```python
from build123d import *

# Parameters (mm, degrees)
SKETCH1_R           = 5
BOSS_EXTRUDE1_DEPTH = 2
SKETCH2_R           = 4.3
BOSS_EXTRUDE2_DEPTH = 3
CHAMFER1_SIZE       = 1
CHAMFER1_SIZE2      = 0.577350269


with BuildPart() as part:
    # Sketch1 → Boss-Extrude1 (new body)
    with BuildSketch(Plane(origin=(0, 0, 0), x_dir=(1, 0, 0), z_dir=(0, 1, 0))):
        Circle(SKETCH1_R)
    extrude(amount=BOSS_EXTRUDE1_DEPTH)

    # Sketch2 → Boss-Extrude2 (add)
    with BuildSketch(Plane(origin=(0, 2, 0), x_dir=(1, 0, 0), z_dir=(0, 1, 0))):
        Circle(SKETCH2_R)
    extrude(amount=BOSS_EXTRUDE2_DEPTH)

    # Chamfer1
    chamfer1_edges = [part.edges().sort_by_distance(p)[0] for p in [
        (-4.3, 5, 0),
    ]]
    chamfer1_side = [part.faces().sort_by_distance(p)[0] for p in [
        (-4.3, 3.5, 0),
    ]]
    chamfer(chamfer1_edges, length=CHAMFER1_SIZE, length2=CHAMFER1_SIZE2, reference=chamfer1_side[0])


solid = part.part
```
Read the model definition and answer for the solid it produces. Units are mm, in the model's axes. A direction names the side the tool comes from. Give positions to 0.01 mm unless a question says otherwise; leave off trailing zeros. Write each loop counter-clockwise with the first axis right and the second up, starting at its lowest first coordinate (ties: lowest second). Pieces come first, ordered by that corner, then holes. Notation, with made-up numbers: M 72,57.25 L 77,57.25 A17 cw 77,84.25 Z; hole C -9,82.25 d8. An arc over 180 degrees is marked long. Put each result on its own line as item: value. Start each with the question number.
1. Consider line 1 along Y through (x, z) = (-2.5, 4); line 2 along X through (y, z) = (4.6, 0); line 3 along Z through (x, y) = (-1.75, 3.1). Determine where each line is inside the solid, lowest interval first.
2. Which of the six approach directions +Z, -Z, +X, -X, +Y, -Y give full straight-line access (tool end or side, diameter ignored) to faces 1 (the flat face through (0, 5, 0)), 2 (the flat face through (2, 2, -4))?
3. The part is cut by section C-C, the plane y = 3. Give the vertices of the cut face in (x, z).
4. This flat-tipped pin is pushed along its axis until it touches: pin 1 Ø3 at (y, z) = (4, -1) entering from +X. Where does it stop, or does it pass through?
5. The part is cut by section D-D, the plane y = 1.8. Give the vertices of the cut face in (x, z), and give its area (3 significant figures).
6. The part is cut by section B-B, the plane x = 0. Give the vertices of the cut face in (y, z), and give its area (3 significant figures).
7. The part is cut by section A-A, the plane z = 0. Give the vertices of the cut face in (x, y).
Final values:
1. line 1: y = 0 to 2
1. line 2: x = -3.95 to 3.95
1. line 3: z = -3.93 to 3.93
2. face 1: +Z, -Z, +X, -X, +Y
2. face 2: +Y
3. outline: C 0,0 d8.6
4. pin 1: stops at x = 4.3
5. outline: C 0,0 d10
5. area: 78.5 mm²
6. outline: M 0,-5 L 2,-5 L 2,-4.3 L 4,-4.3 L 5,-3.72 L 5,3.72 L 4,4.3 L 2,4.3 L 2,5 L 0,5 Z
6. area: 45.2 mm²
7. outline: M -5,0 L 5,0 L 5,2 L 4.3,2 L 4.3,4 L 3.72,5 L -3.72,5 L -4.3,4 L -4.3,2 L -5,2 Z
